Build history of the part. All positions in model axes, mm. Face numbers are marked on the shaded views. A direction names the side the tool comes from. Give positions to 0.01 mm unless a question says otherwise; leave off trailing zeros. Order: outer loops, then holes, each group sorted by start corner. A loop starts at its lowest first (then second) coordinate and runs counter-clockwise, first axis right, second up. Notation, with made-up numbers: (-40, 28.25) - (-5, 28.25) arc R34 cw to (-5, 58.25) - close; hole circle Ø4 at (9.5, -1.5). An arc over 180 degrees is marked (long way). Use a Markdown table: item, result.
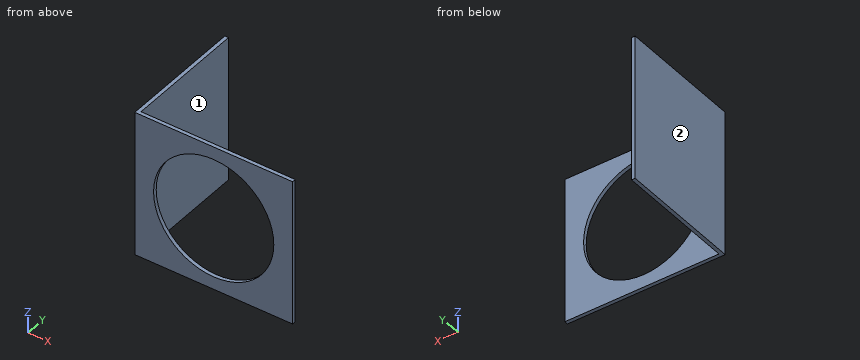
Autodesk Inventor part; units mm, degrees
ref_plane "YZ Plane" through (0, 0, 0) normal (1, 0, 0) x (0, 1, 0)
ref_plane "XZ Plane" through (0, 0, 0) normal (0, 1, 0) x (-1, 0, 0)
ref_plane "XY Plane" through (0, 0, 0) normal (0, 0, 1) x (1, 0, 0)
sketch "Sketch1" plane through (0, 0, 0) normal (0, 1, 0) x (-1, 0, 0)
  circle A0 centre (0, 0) radius 49.5
  line L0 (65, 60) -> (-65, 60)
  line L1 (-65, 60) -> (-65, -60)
  line L2 (-65, -60) -> (65, -60)
  line L3 (65, -60) -> (65, 60)
  line L4 (65, 60) -> (-65, -60) construction
  line L5 (-65, 60) -> (65, -60) construction
  dimension "d0" = 99
  dimension "d1" = 130
  dimension "d2" = 120
extrude "Extrusion1" add sketch "Sketch1" along normal blind 3
sketch "Sketch2" plane through (0, 3, 0) normal (0, 1, 0) x (1, 0, 0)
  line L0 (-65, -60) -> (-62, -60)
  line L1 (-62, -60) -> (-62, 60)
  line L2 (-62, 60) -> (-65, 60)
  line L3 (-65, 60) -> (-65, -60)
  line L4 (-65, -60) -> (-62, 60) construction
  line L5 (-62, -60) -> (-65, 60) construction
  line L6 (-65, 60) -> (-65, -60)
  point P0 (0, 0)
  point P1 (-63.5, 0)
  point P2 (-65, 0)
  dimension "d5" = 3
  dimension "d6" = 120
extrude "Extrusion2" add sketch "Sketch2" along normal blind 100
properties part number "ammonia filter bracket"
1) Slice it at D-D (z = -13). Write the cut outline in (x, y).
Computed:
| item | result |
|---|---|
| outline | (-65, 0) - (-47.76, 0) - (-47.76, 3) - (-62, 3) - (-62, 103) - (-65, 103) - close; (47.76, 0) - (65, 0) - (65, 3) - (47.76, 3) - close |
2) Slice it at A-A (z = 0). Write the cut outline in (x, y).
Computed:
| item | result |
|---|---|
| outline | (-65, 0) - (-49.5, 0) - (-49.5, 3) - (-62, 3) - (-62, 103) - (-65, 103) - close; (49.5, 0) - (65, 0) - (65, 3) - (49.5, 3) - close |
3) Wall check: line 1 (Z direction, x = 0, y = 1.25); line 2 (X direction, y = 61, z = -36); line 3 (Y direction, x = 58, z = -26.5). Give the ranges that are in metal, low to high. Write a range as from..to.
Computed:
| item | result |
|---|---|
| line 1 | z = -60..-49.5, 49.5..60 |
| line 2 | x = -65..-62 |
| line 3 | y = 0..3 |
4) Pin check, flat tips, straight feed: P1, Ø5, axis at y = 72.5, z = 43.5, coming from the +X side; P2, Ø6, axis at x = -36.5, z = 26.5, coming from the +Y side (1 decimal); P3, Ø5, axis at x = 33, z = -35.5, coming from the +Y side; P4, Ø1.5, axis at x = 43.5, z = -42, coming from the -Y side. Stop position of each tip, or through.
Computed:
| item | result |
|---|---|
| P1 | stops at x = -62 |
| P2 | passes through |
| P3 | stops at y = 3 |
| P4 | stops at y = 0 |
5) Slice it at C-C (y = 51). Write the cut outline in (x, z).
Computed:
| item | result |
|---|---|
| outline | (-65, -60) - (-62, -60) - (-62, 60) - (-65, 60) - close |
6) Slice it at B-B (x = 0). Write the cut outline in (y, z).
Computed:
| item | result |
|---|---|
| outline | (0, -60) - (3, -60) - (3, -49.5) - (0, -49.5) - close; (0, 49.5) - (3, 49.5) - (3, 60) - (0, 60) - close |
7) Tool access for the marked faces 1 and 2: list every direction of +Z, -Z, +X, -X, +Y, -Y with a clear straight run to the whole face (end or side of a thin tool).
Computed:
| item | result |
|---|---|
| face 1 | +Z, -Z, +X, +Y |
| face 2 | +Z, -Z, -X, +Y, -Y |
